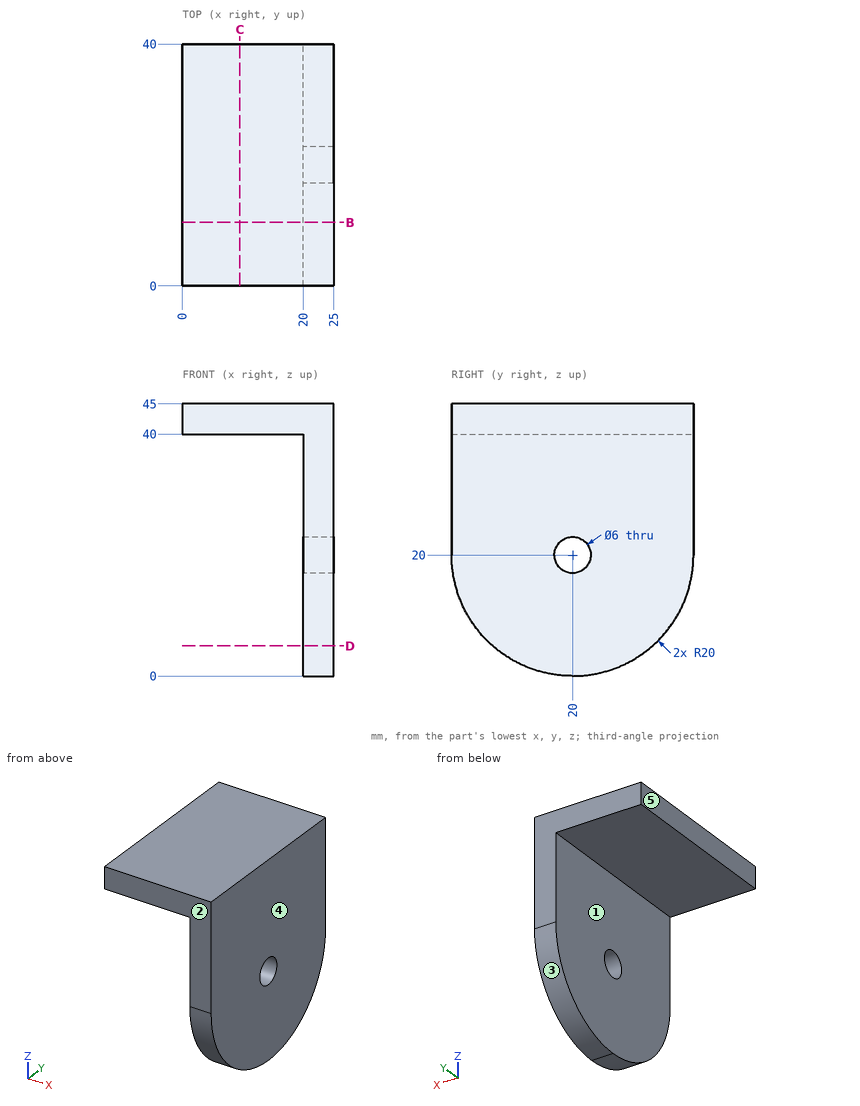
Geometry check sheet. Reference: drawing and pictorial views, mm from the part's lowest x, y, z. A direction names the side the tool comes from. Round coordinates to 2 decimals unless told otherwise and drop trailing zeros. Write each loop counter-clockwise with the first axis right and the second up, starting at its lowest first coordinate (ties: lowest second). Pieces come first, ordered by that corner, then holes. Notation, with made-up numbers: (58.5, 73.5) -> (104.5, 73.5) arc R14 ccw to (104.5, 88.5) -> close; hole circle Ø3 at (59, 74.25). An arc over 180 degrees is marked (long way). Answer as CSV lines item,"result". Start each with the question number.
1) Section check D-D on z = 5. Enter the section's corners in (x, y).
2) Section check B-B on y = 10.5. Enter the section's corners in (x, z).
3) Go/stop test with flat-tipped pins: P1, Ø1.5, axis at x = 16, y = 9, coming from the -Z side; P2, Ø6, axis at x = 17.5, z = 5.5, coming from the -Y side. Record where each tip stops, or that it passes through.
4) Release check for a two-part mould opening along X. For the marked faces 3, 4 and 5 record: pulls with the +X half, pulls with the -X half, needs draft (parallel to the pull), parting line crosses it, or undercut.
5) Tool access check on the marked faces 1 and 2. Record the directions out of +Z, -Z, +X, -X, +Y, -Y that give a thin tool (end or side, any length) a straight path to the whole face; none if there is none.
6) Section check C-C on x = 9.5. Enter the section's corners in (y, z), and give its area (3 significant figures).
7) Material ranges on line 1 (Y direction, x = 23.6, z = 20); line 2 (X direction, y = 38, z = 28.5); line 3 (Z direction, x = 9.25, y = 21), recorded low to high. Write a range as from..to.
Found:
1,outline,"(20, 6.77) -> (25, 6.77) -> (25, 33.23) -> (20, 33.23) -> close"
2,outline,"(0, 40) -> (20, 40) -> (20, 2.4) -> (25, 2.4) -> (25, 45) -> (0, 45) -> close"
3,P1,"stops at z = 40"
3,P2,"stops at y = 4.67"
4,face 3,"needs draft"
4,face 4,"pulls with the +X half"
4,face 5,"pulls with the -X half"
5,face 1,"-Z, -X, +Y, -Y"
5,face 2,"+Z, -Z, +X, -X, -Y"
6,outline,"(0, 40) -> (40, 40) -> (40, 45) -> (0, 45) -> close"
6,area,"200 mm^2"
7,line 1,"y = 0..17, 23..40"
7,line 2,"x = 20..25"
7,line 3,"z = 40..45"
